from build123d import *

# Parameters (mm, degrees)
BOSS_EXTRUDE1_DEPTH = 1.4605
SKETCH2_W           = 2.921
SKETCH2_H           = 25.4
SKETCH2_H_2         = 12.7
CUT_EXTRUDE1_DEPTH  = 2.921
SKETCH3_W           = 6.35
SKETCH3_H           = 2.921
BOSS_EXTRUDE2_DEPTH = 6.0452
CUT_EXTRUDE2_DEPTH  = 147.066332108


with BuildPart() as part:
    # Sketch1 → Boss-Extrude1 (new, symmetric)
    with BuildSketch(Plane.XY):
        Polygon((-36.517931963, 109.22), (36.517931963, 137.255841429), (36.517931963, -109.22), (-36.517931963, -109.22), align=None)
    extrude(amount=BOSS_EXTRUDE1_DEPTH, both=True)

    # Sketch2 → Cut-Extrude1 (cut)
    with BuildSketch(Plane.XY.offset(1.4605)):
        with Locations((-35.057431963, -96.52)):
            Rectangle(SKETCH2_W, SKETCH2_H)
        with Locations((-35.057431963, -45.72)):
            Rectangle(SKETCH2_W, SKETCH2_H)
        with Locations((-35.057431963, 5.08)):
            Rectangle(SKETCH2_W, SKETCH2_H)
        with Locations((-35.057431963, 49.53)):
            Rectangle(SKETCH2_W, SKETCH2_H_2)
        with Locations((35.057431963, 49.53)):
            Rectangle(SKETCH2_W, SKETCH2_H_2)
        with Locations((35.057431963, 5.08)):
            Rectangle(SKETCH2_W, SKETCH2_H)
        with Locations((35.057431963, -96.52)):
            Rectangle(SKETCH2_W, SKETCH2_H)
        with Locations((35.057431963, -45.72)):
            Rectangle(SKETCH2_W, SKETCH2_H)
        with Locations((35.057431963, 62.23)):
            Rectangle(SKETCH2_W, SKETCH2_H_2)
    extrude(amount=-CUT_EXTRUDE1_DEPTH, mode=Mode.SUBTRACT)

    # Sketch3 → Boss-Extrude2 (add)
    with BuildSketch(Plane(origin=(-41.231132307, 107.410771898, 0), x_dir=(0.9335804264972012, 0.35836794954530177, 0), z_dir=(-0.35836794954530177, 0.9335804264972012, 0))):
        with Locations((75.914520953, 0)):
            Rectangle(SKETCH3_W, SKETCH3_H)
        with Locations((63.214520953, 0)):
            Rectangle(SKETCH3_W, SKETCH3_H)
        with Locations((50.514520953, 0)):
            Rectangle(SKETCH3_W, SKETCH3_H)
        with Locations((37.814520953, 0)):
            Rectangle(SKETCH3_W, SKETCH3_H)
        with Locations((25.114520953, 0)):
            Rectangle(SKETCH3_W, SKETCH3_H)
        with Locations((12.414520953, 0)):
            Rectangle(SKETCH3_W, SKETCH3_H)
    extrude(amount=BOSS_EXTRUDE2_DEPTH)

    # Sketch5 → Cut-Extrude2 (cut, through all)
    with BuildSketch(Plane.XY.offset(1.4605)):
        Polygon((-15.875, 52.374079158), (-8.001, 55.39662457), (-8.001, -98.27337543), (-15.875, -101.295920842), align=None)
        Polygon((8.001, 61.539216859), (15.875, 64.561762271), (15.875, -89.108237729), (8.001, -92.130783141), align=None)
    extrude(amount=-CUT_EXTRUDE2_DEPTH, mode=Mode.SUBTRACT)


solid = part.part
Part model, mm, in its own coordinate system. Give positions to 0.01 mm unless a question says otherwise; leave off trailing zeros. Write each loop counter-clockwise with the first axis right and the second up, starting at its lowest first coordinate (ties: lowest second). Pieces come first, ordered by that corner, then holes.
1) Pin check, flat tips, straight feed: pin 1 (1.5 mm diameter, centred on y = 13, z = -0.5, fed in from -X); pin 2 (0.9 mm diameter, centred on x = 34.5, z = -0.5, fed in from +Y); pin 3 (0.9 mm diameter, centred on x = 35, z = 0.5, fed in from -Y). Stop position of each tip, or through.
Resolved:
pin 1: stops at x = -33.6
pin 2: stops at y = 136.65
pin 3: stops at y = -83.82
2) Cut at A-A on y = 40.5. Write the cut outline in (x, z) (1 decimal).
Resolved:
outline: (-36.5, -1.5) - (-15.9, -1.5) - (-15.9, 1.5) - (-36.5, 1.5) - close; (-8, -1.5) - (8, -1.5) - (8, 1.5) - (-8, 1.5) - close; (15.9, -1.5) - (36.5, -1.5) - (36.5, 1.5) - (15.9, 1.5) - close
3) Cut at B-B on z = -0.05. State how many separate pieces and enclosed holes the cut face has, then the cut area to 3 significant figures.
Resolved:
separate pieces: 1
enclosed holes: 2
area: 14,200 mm2
4) Probe L1, parallel to X at y = -85, z = 0.25 (3 decimals); L2, parallel to X at y = -13.5, z = 1.1 (3 decimals); L3, parallel to X at y = -96, z = 0.8 (3 decimals). List the from-to ranges inside material, lowest first.
Resolved:
L1: x = -33.597 to -15.875, -8.001 to 8.001, 15.875 to 33.597
L2: x = -36.518 to -15.875, -8.001 to 8.001, 15.875 to 36.518
L3: x = -33.597 to -15.875, -8.001 to 33.597
